Build history of the part. All positions in model axes, mm. A direction names the side the tool comes from. Give positions to 0.01 mm unless a question says otherwise; leave off trailing zeros. Order: outer loops, then holes, each group sorted by start corner. A loop starts at its lowest first (then second) coordinate and runs counter-clockwise, first axis right, second up. Notation, with made-up numbers: M 41,31 L 88,31 A19 cw 88,53 Z; hole C 87,75.5 d7. An arc over 180 degrees is marked long. Answer as CSV lines item,"result".
from build123d import *

# Parameters (mm, degrees)
F1_DEPTH = 50.8
F3_DEPTH = 6.35
F5_DEPTH = 12.7
F7_DEPTH = 76.2
F8_R     = 12.7


with BuildPart() as f1:
    # F0 (on Front) → F1 (new body)
    with BuildSketch(Plane.XZ):
        Polygon((0, 38.1), (0, 0), (76.2, 0), (76.2, 12.7), (50.8, 12.7), (50.8, 38.1), (38.1, 38.1), (38.1, 50.8), (12.7, 50.8), align=None)
    extrude(amount=F1_DEPTH)

    # F2 (on face) → F3 (cut, symmetric)
    with BuildSketch(Plane.XZ.offset(50.8)):
        Polygon((38.1, 50.8), (25.4, 50.8), (25.4, 25.4), (50.8, 25.4), (50.8, 38.1), (38.1, 38.1), align=None)
    extrude(amount=F3_DEPTH, both=True, mode=Mode.SUBTRACT)

    # F4 (on face) → F5 (cut)
    with BuildSketch(Plane(origin=(0, 0, 0), x_dir=(-1, 0, 0), z_dir=(0, 1, 0))):
        Polygon((-25.4, 25.4), (-25.4, 50.8), (-38.1, 50.8), (-38.1, 38.1), (-50.8, 38.1), (-50.8, 25.4), align=None)
    extrude(amount=-F5_DEPTH, mode=Mode.SUBTRACT)

    # F6 (on face) → F7 (cut)
    with BuildSketch(Plane.YZ.offset(76.2)):
        with BuildLine():
            Line((-28.575, 12.7), (-22.225, 12.7))
            ThreePointArc((-22.225, 12.7), (-25.4, 15.875), (-28.575, 12.7))
        make_face()
        with BuildLine():
            ThreePointArc((-28.575, 12.7), (-25.4, 9.525), (-22.225, 12.7))
            Line((-22.225, 12.7), (-28.575, 12.7))
        make_face()
    extrude(amount=-F7_DEPTH, mode=Mode.SUBTRACT)

    # F8
    f8_edges = [f1.edges().sort_by_distance(p)[0] for p in [
        (76.2, -50.8, 6.35),
        (76.2, 0, 6.35),
    ]]
    fillet(f8_edges, radius=F8_R)


solid = f1.part
Item 1: Band-saw the part on B-B (x = 48). Give the cut face in (y, z) (3 decimals).
Geometry says:
outline,"M -50.8,0 L 0,0 L 0,25.4 L -12.7,25.4 L -12.7,38.1 L -44.45,38.1 L -44.45,25.4 L -50.8,25.4 Z; hole C -25.4,12.7 d6.35"
Item 2: Probe line 1 along Z through (x, y) = (71, -21); line 2 along X through (y, z) = (-35, 16); line 3 along Y through (x, z) = (44.5, 12.7) (3 decimals). List the from-to ranges inside material, lowest first. Write a range as from..to.
Geometry says:
line 1,"z = 0..12.7"
line 2,"x = 0..50.8"
line 3,"y = -50.8..-28.575, -22.225..0"
Item 3: Band-saw the part on C-C (z = 14). Give the cut face in (x, y), and give its area (3 significant figures).
Geometry says:
outline,"M 0,-50.8 L 50.8,-50.8 L 50.8,-28.3 L 0,-28.3 Z; M 0,-22.5 L 50.8,-22.5 L 50.8,0 L 0,0 Z"
area,"2,290 mm2"
Item 4: Band-saw the part on A-A (y = -25.4). Give the cut face in (x, z) (3 decimals), and give its area (3 significant figures).
Geometry says:
outline,"M 0,0 L 76.2,0 L 76.2,9.525 L 0,9.525 Z; M 0,15.875 L 50.8,15.875 L 50.8,38.1 L 38.1,38.1 L 38.1,50.8 L 12.7,50.8 L 0,38.1 Z"
area,"2,260 mm2"
Item 5: Band-saw the part on D-D (z = 37). Give the cut face in (x, y).
Geometry says:
outline,"M 0,-50.8 L 25.4,-50.8 L 25.4,-44.45 L 50.8,-44.45 L 50.8,-12.7 L 25.4,-12.7 L 25.4,0 L 0,0 Z"
Item 6: 3-axis set-ups, long thin cutter, end or side, ignore diameter. For faces 1 (the flat face through (35, -44.45, 35)), 2 (the flat face through (35, -12.7, 35)), 3 (the flat face through (45, -28, 38.1)), 4 (the flat face through (38, -25, 0)): which of +Z, -Z, +X, -X, +Y, -Y reach the whole face in a straight line?
Geometry says:
face 1,"+Z, +X, -Y"
face 2,"+Z, +X, +Y"
face 3,"+Z, +X, +Y, -Y"
face 4,"-Z, +X, -X, +Y, -Y"
Item 7: Drop flat-ended pins along their axis: pin 1 (4 mm diameter, centred on x = 62.5, y = -29.5, fed in from +Z); pin 2 (7 mm diameter, centred on y = -47.5, z = 35.5, fed in from +X); pin 3 (5 mm diameter, centred on x = 42, y = -47.5, fed in from +Z). Give the stop position or say it passes through.
Geometry says:
pin 1,"stops at z = 12.7"
pin 2,"stops at x = 50.8"
pin 3,"stops at z = 25.4"
